Verification items for this drawing (mm, ordinates from the low corner). Give positions to 0.01 mm unless a question says otherwise; leave off trailing zeros. Loops run counter-clockwise (first coordinate to the right, second up) from the corner with the lowest first, then second, coordinate; pieces in that order, holes last. Notation, with made-up numbers: (69.5, 89) -> (81.5, 89) arc R21 cw to (81.5, 127) -> close; hole circle Ø5 at (11.5, 59). An arc over 180 degrees is marked (long way). Answer as a JSON object with one key per item and string values.
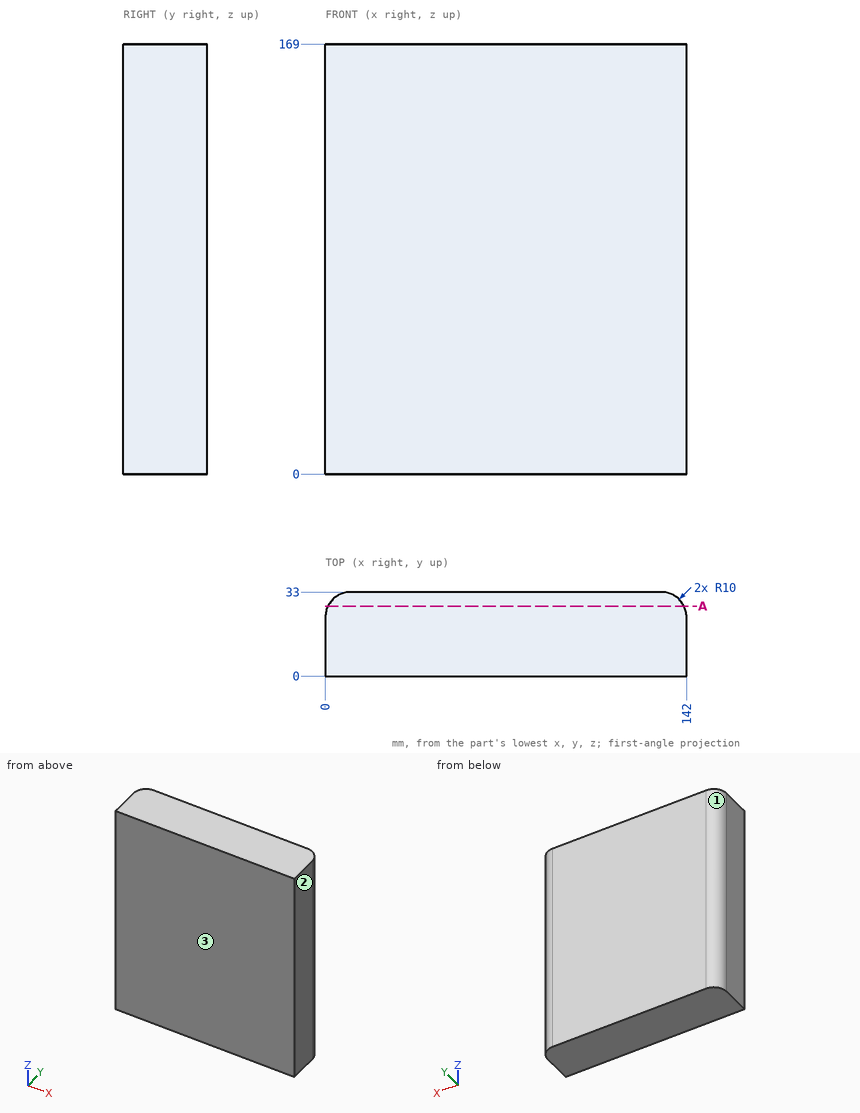
1) Material ranges on line 1 along X through (y, z) = (24.5, 100); line 2 along Y through (x, z) = (7, 155); line 3 along X through (y, z) = (28.5, 129), recorded low to high. Write a range as from..to.
Geometry check:
{"line 1": "x = 0.11..141.89", "line 2": "y = 0..32.54", "line 3": "x = 1.65..140.35"}
2) Section check A-A on y = 27.5. Record the cut outline in (x, z).
Geometry check:
{"outline": "(1.07, 0) -> (140.93, 0) -> (140.93, 169) -> (1.07, 169) -> close"}
3) Depth check by flat-ended pin: P1, Ø2, axis at y = 27.5, z = 29, coming from the +X side. Enter the tip coordinate at first touch or a pass-through.
Geometry check:
{"P1": "stops at x = 141.37"}
4) Draft check along Y on the marked faces 1, 2 and 3. Enter one of: pulls with the +Y half, pulls with the -Y half, needs draft (parallel to the pull), parting line crosses it, or undercut.
Geometry check:
{"face 1": "pulls with the +Y half", "face 2": "needs draft", "face 3": "pulls with the -Y half"}
